Geometry check sheet. Reference: the model listing, model coordinates, mm. A direction names the side the tool comes from. Coordinates: 2 decimals unless noted, no trailing zeros. Write each loop counter-clockwise with the first axis right and the second up, starting at its lowest first coordinate (ties: lowest second). Pieces come first, ordered by that corner, then holes. Notation, with made-up numbers: M 52,-9 L 74,-9 A11 ccw 74,-5 Z; hole C 15.25,75 d5. An arc over 180 degrees is marked long. Write each question's results on one line, items separated by ' | '.
```python
from build123d import *

# Parameters (mm, degrees)
F0_W     = 45.83
F0_H     = 34
F1_DEPTH = 3
F2_W     = 36.04
F2_H     = 29.03
F3_DEPTH = 0.6
F2_W_2   = 2.711302
F2_H_2   = 22.891694
F4_DEPTH = 1.1


with BuildPart() as f1:
    # F0 (on Top) → F1 (new body)
    with BuildSketch(Plane.XY):
        Rectangle(F0_W, F0_H)
    extrude(amount=F1_DEPTH)

    # F2 (on face) → F3 (cut)
    with BuildSketch(Plane.XY.offset(3)):
        Polygon((20.203698, 15.784912), (-21.650197, 15.784912), (-21.650197, -15.8541), (20.203698, -15.8541), (20.203698, -11.445847), (20.203698, 11.445847), align=None)
        with Locations((-2.605, 0.008636)):
            Rectangle(F2_W, F2_H, mode=Mode.SUBTRACT)
    extrude(amount=-F3_DEPTH, mode=Mode.SUBTRACT)

    # F2 (on face) → F4 (cut)
    with BuildSketch(Plane.XY.offset(3)):
        with Locations((21.559349, 0)):
            Rectangle(F2_W_2, F2_H_2)
    extrude(amount=-F4_DEPTH, mode=Mode.SUBTRACT)


with BuildPart() as f5_1:
    # F5: copy of F1
    add(f1.part)


solid = f5_1.part
```
Q1. Sectioned sample at A-A on x = 19.5. Record the cut outline in (y, z).
Geometry check:
outline: M -17,0 L 17,0 L 17,3 L 15.78,3 L 15.78,2.4 L -15.85,2.4 L -15.85,3 L -17,3 Z
Q2. Sectioned sample at B-B on y = 12.5. Record the cut outline in (x, z) (3 decimals).
Geometry check:
outline: M -22.915,0 L 22.915,0 L 22.915,3 L 20.204,3 L 20.204,2.4 L 15.415,2.4 L 15.415,3 L -20.625,3 L -20.625,2.4 L -21.65,2.4 L -21.65,3 L -22.915,3 Z
Q3. Depth check by flat-ended pin: P1, Ø3, axis at x = 21.5, y = 3, coming from the +Z side; P2, Ø0.7, axis at y = -6, z = 3, coming from the +X side (3 decimals). Enter the tip coordinate at first touch or a pass-through.
Geometry check:
P1: stops at z = 2.4 | P2: stops at x = 15.415
Q4. Access from +Z, -Z, +X, -X, +Y, -Y to the whole of each face (thin tool, end or side, straight path). Record for faces 4 (the flat face through (0, 17, 1)), 5 (the flat face through (21.5, -11.446, 2.5)).
Geometry check:
face 4: +Z, -Z, +X, -X, +Y | face 5: +Z, +X
Q5. Sectioned sample at C-C on x = -3.5. Record the cut outline in (y, z), and give its area (3 significant figures).
Geometry check:
outline: M -17,0 L 17,0 L 17,3 L 15.78,3 L 15.78,2.4 L 14.52,2.4 L 14.52,3 L -14.51,3 L -14.51,2.4 L -15.85,2.4 L -15.85,3 L -17,3 Z | area: 100 mm2
Q6. Scan lines: probe 1 along Y at (x, z) = (-14.5, 2.85); probe 2 along Z at (x, y) = (-18, 15); probe 3 along X at (y, z) = (2.5, 2.75) (3 decimals). Record each from-to range of solid material in increasing order.
Geometry check:
probe 1: y = -17 to -15.85, -14.51 to 14.52, 15.78 to 17 | probe 2: z = 0 to 2.4 | probe 3: x = -22.915 to -21.65, -20.625 to 15.415
Q7. Mould release check, pull along Y, two halves, no side actions. Record for faces 1 (the flat face through (-22.915, 0, 1)), 2 (the flat face through (0, -17, 1)), 3 (the flat face through (21.5, 11.446, 2.5)): pulls with the +Y half, pulls with the -Y half, needs draft (parallel to the pull), parting line crosses it, or undercut.
Geometry check:
face 1: needs draft | face 2: pulls with the -Y half | face 3: undercut
